For this review, take the finished solid that the model builds, in its own axes (mm). A direction names the side the tool comes from. Round coordinates to 2 decimals unless told otherwise and drop trailing zeros.
Autodesk Inventor part; units mm, degrees
ref_plane "to_bolt_XY" through (5, -8, 0) normal (1, 0, 0) x (0, 0, -1)
ref_plane "to_bolt_YZ" through (5, -8, 0) normal (0, 0, -1) x (0, 1, 0)
ref_plane "to_bolt_ZX" through (5, -8, 0) normal (0, 1, 0) x (1, 0, 0)
sketch "Sketch_14" plane through (0, 0, 0) normal (1, 0, 0) x (0, 1, 0)
  line L0 (0, -5) -> (0, 5)
  line L1 (0, 5) -> (12, 5)
  line L2 (12, 5) -> (12.5, 4.5)
  line L3 (12.5, 4.5) -> (12.5, -4.5)
  line L4 (12.5, -4.5) -> (12, -5)
  line L5 (12, -5) -> (0, -5)
  line L6 (0, -5) -> (0, 5)
revolve "Revolution1" add sketch "Sketch_14" angle 360 about axis through (0, 0, -5) along (0, 0, -1)
sketch "Sketch_15" plane through (0, 0, 0) normal (1, 0, 0) x (0, 1, 0)
  line L0 (0, -5) -> (0, 5)
  line L1 (0, 5) -> (4.5, 5)
  line L2 (4.5, 5) -> (4, 4.5)
  line L3 (4, 4.5) -> (4, -4.5)
  line L4 (4, -4.5) -> (4.5, -5)
  line L5 (4.5, -5) -> (0, -5)
  line L6 (0, -5) -> (0, 5)
revolve "Revolution2" cut sketch "Sketch_15" angle 360 about axis through (0, 0, -5) along (0, 0, -1)
sketch "Sketch_16" plane through (0, 0, 0) normal (0, 0, 1) x (1, 0, 0)
  arc A0 (-0.75, -13.4792) -> (0.75, -13.4792) centre (0, 0) ccw
  line L0 (0.75, -13.4792) -> (0.75, 0)
  line L1 (0.75, 0) -> (-0.75, 0)
  line L2 (-0.75, 0) -> (-0.75, -13.4792)
extrude "Extrusion1" cut sketch "Sketch_16" along normal mid plane 10
sketch "Sketch_18" plane through (9, 0, 0) normal (1, 0, 0) x (0, 0, -1)
  line L0 (5, 0) -> (-5, 0)
  line L1 (-5, 0) -> (-5, 2)
  line L2 (-5, 2) -> (-4.621, 1.621)
  line L3 (-4.621, 1.621) -> (4.621, 1.621)
  line L4 (4.621, 1.621) -> (5, 2)
  line L5 (5, 2) -> (5, 0)
  line L6 (5, 0) -> (-5, 0)
revolve "Revolution3" cut sketch "Sketch_18" angle 360 about axis through (9, 0, -5) along (0, 0, -1)
thread "Thread1"
sketch "Sketch_20" plane through (-9, 0, 0) normal (1, 0, 0) x (0, 0, -1)
  line L0 (5, 0) -> (-5, 0)
  line L1 (-5, 0) -> (-5, 2)
  line L2 (-5, 2) -> (-4.621, 1.621)
  line L3 (-4.621, 1.621) -> (4.621, 1.621)
  line L4 (4.621, 1.621) -> (5, 2)
  line L5 (5, 2) -> (5, 0)
  line L6 (5, 0) -> (-5, 0)
revolve "Revolution4" cut sketch "Sketch_20" angle 360 about axis through (-9, 0, -5) along (0, 0, -1)
thread "Thread2"
sketch "Sketch_22" plane through (0, 9, 0) normal (0, 1, 0) x (1, 0, 0)
  line L0 (0, 5) -> (0, -5)
  line L1 (0, -5) -> (-2, -5)
  line L2 (-2, -5) -> (-1.621, -4.621)
  line L3 (-1.621, -4.621) -> (-1.621, 4.621)
  line L4 (-1.621, 4.621) -> (-2, 5)
  line L5 (-2, 5) -> (0, 5)
  line L6 (0, 5) -> (0, -5)
revolve "Revolution5" cut sketch "Sketch_22" angle 360 about axis through (0, 9, -5) along (0, 0, -1)
thread "Thread3"
sketch "Sketch_23" plane through (0, -8, 0) normal (0, 1, 0) x (1, 0, 0)
  line L0 (12.5, 0) -> (0, 0)
  line L1 (0, 0) -> (0, 2.25)
  line L2 (0, 2.25) -> (5, 2.25)
  line L3 (5, 2.25) -> (5, 3.75)
  line L4 (5, 3.75) -> (12.5, 3.75)
  line L5 (12.5, 3.75) -> (12.5, 0)
  line L6 (12.5, 0) -> (0, 0)
revolve "Revolution6" cut sketch "Sketch_23" angle 360 about axis through (12.5, -8, 0) along (1, 0, 0)
sketch "Sketch_25" plane through (0, 0, 0) normal (0, 0, 1) x (1, 0, 0)
  line L0 (-0.75, -8) -> (-10.9659, -8)
  line L1 (-10.9659, -8) -> (-10.9659, -6.379)
  line L2 (-10.9659, -6.379) -> (-1.129, -6.379)
  line L3 (-1.129, -6.379) -> (-0.75, -6)
  line L4 (-0.75, -6) -> (-0.75, -8)
  line L5 (-0.75, -8) -> (-10.9659, -8)
revolve "Revolution7" cut sketch "Sketch_25" angle 360 about axis through (-0.75, -8, 0) along (1, 0, 0)
thread "Thread4"
ref_plane "to_bolt_XY" through (5, -8, 0) normal (1, 0, 0) x (0, 0, -1)
ref_plane "to_bolt_YZ" through (5, -8, 0) normal (0, 0, -1) x (0, 1, 0)
ref_plane "to_bolt_ZX" through (5, -8, 0) normal (0, 1, 0) x (1, 0, 0)
properties part number "SCSTR8-10b" material "鋼、炭素鋼"
(1) Wall thickness on L1, parallel to X at y = 0, z = 0.25; L2, parallel to Y at x = 0, z = -2.5; L3, parallel to Y at x = 2.85, z = 0: over which ranges is each line inside the solid? List them lowest first.
(2) Add section A-A on y = 0. Count the separate pieces of the cut face and the enclosed holes in it, plus the area to 3 significant figures.
(3) Clearance check with flat-ended pins moving along their axes: P1, Ø5, axis at y = 4, z = -1.5, coming from the +X side; P2, Ø2, axis at y = 9, z = 2.5, coming from the +X side; P3, Ø6, axis at x = -8, z = -2.5, coming from the -Y side; P4, Ø1.9, axis at y = -8, z = 0, coming from the -X side. State where each tip first meets the part, or that it passes through.
(4) Tool access review of faces 5 (the face through (7.674, -4.253, -0.144)), 6 (the face through (-0.75, -10, -1)), 7 (the face through (10.607, -0.211, -0.065)): name each direction out of +Z, -Z, +X, -X, +Y, -Y from which nothing blocks a thin tool from reaching the whole face with its end or side.
(5) Draft analysis for pull direction Z (two halves, no side actions). For faces 1 (the face through (0.211, 10.607, -0.065)), 2 (the face through (2.9, -5.77, 0.29)), 3 (the face through (-0.52, 12.13, 4.86)), 4 (the face through (-5, 0, -5)), state which applies: pulls with the +Z half, pulls with the -Z half, needs draft (parallel to the pull), parting line crosses it, or undercut.
Here are the results:
1. L1: x = -12.5 to -10.62, -7.38 to -4, 4 to 7.38, 10.62 to 12.5
1. L2: y = 4 to 7.38, 10.62 to 12.5
1. L3: y = -12.17 to -10.25, -5.75 to -2.81, 2.81 to 12.17
2. separate pieces: 4
2. enclosed holes: 0
2. area: 104 mm2
3. P1: stops at x = 12.41
3. P2: stops at x = 9.6
3. P3: stops at y = -11.46
3. P4: passes through
4. face 5: +X
4. face 6: +Z, -Z, -Y
4. face 7: +Z, -Z
5. face 1: needs draft
5. face 2: undercut
5. face 3: pulls with the +Z half
5. face 4: pulls with the -Z half
